```python
from build123d import *

# Parameters (mm, degrees)
BOSS_EXTRUDE1_DEPTH = 2
BOSS_EXTRUDE2_DEPTH = 38
MANUAL_FILLET_DEPTH = 38
SKETCH7_R           = 1.399999999999996
SKETCH7_R_2         = 1.4
SKETCH7_R_3         = 1.3999999999999992
SKETCH7_R_4         = 1.4000000000000026
BOTTOM_SCREWS_DEPTH = 9
LEFT_SCREWS_REACH   = 212.024
SKETCH8_R           = 1.6000000000000127
SKETCH8_R_2         = 1.600000000000008
RIGHT_SCREWS_REACH  = 212.024
SKETCH9_R           = 1.6000000000000127
SKETCH9_R_2         = 1.600000000000007
BOSS_EXTRUDE3_DEPTH = 15
CUT_EXTRUDE1_REACH  = 220.907
SKETCH10_R          = 17.50000000000029
SKETCH10_R_2        = 1.6000000000000194
SKETCH10_R_3        = 1.5999999999999908
CUT_EXTRUDE2_REACH  = 220.907
SKETCH11_R          = 17.500000000000004
SKETCH11_R_2        = 1.600000000000006
SKETCH11_R_3        = 1.5999999999999974
FILLET1_R           = 2


with BuildPart() as part:
    # Sketch2 → Boss-Extrude1 (new body)
    with BuildSketch(Plane.XY):
        Polygon((-113.14018169510446, 0), (113.14018169510446, 2.771e-14), (118.50513169510454, -9.292365980066561), (113.30897927239795, -12.292365980066618), (109.67608007996674, -5.999999999999973), (-109.67608007996674, -6), (-113.30897927239795, -12.292365980066647), (-118.50513169510454, -9.292365980066593), align=None)
    extrude(amount=BOSS_EXTRUDE1_DEPTH)

    # Sketch2<3> → Boss-Extrude2 (add)
    with BuildSketch(Plane.XY):
        Polygon((-113.14018169510446, 0), (113.14018169510446, 2.771e-14), (118.50513169510454, -9.292365980066561), (113.30897927239795, -12.292365980066618), (109.67608007996674, -5.999999999999973), (-109.67608007996674, -6), (-113.30897927239795, -12.292365980066647), (-118.50513169510454, -9.292365980066593), align=None)
    extrude(amount=BOSS_EXTRUDE2_DEPTH)

    # Sketch6 → Manual fillet (add)
    with BuildSketch(Plane(origin=(0, 0, 0), x_dir=(-1, 0, 0), z_dir=(0, 0, -1))):
        with BuildLine():
            Line((-114.87223250267334, -2.99999999999992), (-104.47992765725986, 15.00000000000004))
            ThreePointArc((-104.47992765725986, 15.00000000000004), (-104.47992765725994, 5.00000000000003), (-95.81967361941555, -2.602e-14))
            Line((-95.81967361941555, -2.602e-14), (95.81967361941547, -1.73e-15))
            ThreePointArc((95.81967361941547, -1.73e-15), (104.47992765725988, 5.00000000000004), (104.47992765725981, 15.000000000000083))
            Line((104.47992765725981, 15.000000000000083), (114.87223250267334, -2.999999999999949))
            Line((114.87223250267334, -2.999999999999949), (109.67608007996674, -6))
            Line((109.67608007996674, -6), (-109.67608007996674, -5.999999999999973))
            Line((-109.67608007996674, -5.999999999999973), (-114.87223250267334, -2.99999999999992))
        make_face()
    extrude(amount=-MANUAL_FILLET_DEPTH)

    # Sketch7 → Bottom screws (cut)
    with BuildSketch(Plane.XY):
        with Locations((57.436116251336735, -3.0000000000000004)):
            Circle(SKETCH7_R)
        with Locations((-1.25e-15, -3.0000000000000004)):
            Circle(SKETCH7_R_2)
        with Locations((-57.436116251336564, -3.0000000000000004)):
            Circle(SKETCH7_R)
        with Locations((-28.718058125668286, -3.000000000000001)):
            Circle(SKETCH7_R_3)
        with Locations((28.718058125668367, -3.000000000000001)):
            Circle(SKETCH7_R_3)
        with Locations((-86.15417437700485, -3.000000000000001)):
            Circle(SKETCH7_R_4)
        with Locations((86.15417437700509, -3.000000000000001)):
            Circle(SKETCH7_R_4)
    extrude(amount=BOTTOM_SCREWS_DEPTH, mode=Mode.SUBTRACT)

    # Sketch8 → Left screws (cut, up to next)
    with BuildSketch(Plane(origin=(-79.65898384862079, 45.991135768374306, 0), x_dir=(0, 0, -1), z_dir=(0.8660254037844329, -0.5000000000000101, 0)), mode=Mode.PRIVATE) as left_screws_sk1:
        with Locations(Location((-20, -63.66709165512205, 0), (0, 0, 90))):
            Circle(SKETCH8_R)
    left_screws_tool1 = extrude(left_screws_sk1.sketch, amount=-LEFT_SCREWS_REACH, mode=Mode.PRIVATE) & part.part
    # Sketch8 → Left screws (cut, up to next)
    with BuildSketch(Plane(origin=(-79.65898384862079, 45.991135768374306, 0), x_dir=(0, 0, -1), z_dir=(0.8660254037844329, -0.5000000000000101, 0)), mode=Mode.PRIVATE) as left_screws_sk2:
        with Locations(Location((-4, -63.66709165512205, 0), (0, 0, 90))):
            Circle(SKETCH8_R_2)
    left_screws_tool2 = extrude(left_screws_sk2.sketch, amount=-LEFT_SCREWS_REACH, mode=Mode.PRIVATE) & part.part
    add(left_screws_tool1.solids().sort_by_distance((-111.49253, -9.146183, 20))[0], mode=Mode.SUBTRACT)
    add(left_screws_tool2.solids().sort_by_distance((-111.49253, -9.146183, 4))[0], mode=Mode.SUBTRACT)

    # Sketch9 → Right screws (cut, up to next)
    with BuildSketch(Plane(origin=(79.6589838486208, 45.99113576837435, 0), x_dir=(0, 0, 1), z_dir=(-0.8660254037844329, -0.5000000000000101, 0)), mode=Mode.PRIVATE) as right_screws_sk1:
        with Locations(Location((20, -63.66709165512205, 0), (0, 0, 270))):
            Circle(SKETCH9_R)
    right_screws_tool1 = extrude(right_screws_sk1.sketch, amount=-RIGHT_SCREWS_REACH, mode=Mode.PRIVATE) & part.part
    # Sketch9 → Right screws (cut, up to next)
    with BuildSketch(Plane(origin=(79.6589838486208, 45.99113576837435, 0), x_dir=(0, 0, 1), z_dir=(-0.8660254037844329, -0.5000000000000101, 0)), mode=Mode.PRIVATE) as right_screws_sk2:
        with Locations(Location((4, -63.66709165512205, 0), (0, 0, 270))):
            Circle(SKETCH9_R_2)
    right_screws_tool2 = extrude(right_screws_sk2.sketch, amount=-RIGHT_SCREWS_REACH, mode=Mode.PRIVATE) & part.part
    add(right_screws_tool1.solids().sort_by_distance((111.49253, -9.146183, 20))[0], mode=Mode.SUBTRACT)
    add(right_screws_tool2.solids().sort_by_distance((111.49253, -9.146183, 4))[0], mode=Mode.SUBTRACT)

    # Sketch12 → Boss-Extrude3 (add)
    with BuildSketch(Plane.XY.offset(38.000000000000064)):
        with BuildLine():
            Line((103.86635092950917, 4.062746066806283), (113.30897927239795, -12.292365980066622))
            Line((113.30897927239795, -12.292365980066622), (118.50513169510454, -9.292365980066565))
            Line((118.50513169510454, -9.292365980066565), (104.47992765725988, 15.00000000000004))
            ThreePointArc((104.47992765725988, 15.00000000000004), (105.80397478003607, 9.439883642417866), (103.86635092950917, 4.062746066806283))
        make_face()
        with BuildLine():
            Line((-104.47992765725981, 15.000000000000082), (-118.50513169510454, -9.292365980066597))
            Line((-118.50513169510454, -9.292365980066597), (-113.30897927239795, -12.29236598006665))
            Line((-113.30897927239795, -12.29236598006665), (-103.86635092950914, 4.062746066806313))
            ThreePointArc((-103.86635092950914, 4.062746066806313), (-105.80397478003603, 9.439883642417914), (-104.47992765725981, 15.000000000000082))
        make_face()
    extrude(amount=BOSS_EXTRUDE3_DEPTH)

    # Sketch10 → Cut-Extrude1 (cut, up to next)
    with BuildSketch(Plane(origin=(84.85513627132735, 48.991135768374356, 0), x_dir=(0, 0, -1), z_dir=(0.8660254037844342, 0.500000000000008, 0)), mode=Mode.PRIVATE) as cut_extrude1_sk1:
        with Locations((-38.000000000000085, -76.19999084755334)):
            Circle(SKETCH10_R)
    cut_extrude1_tool1 = extrude(cut_extrude1_sk1.sketch, amount=-CUT_EXTRUDE1_REACH, mode=Mode.PRIVATE) & part.part
    # Sketch10 → Cut-Extrude1 (cut, up to next)
    with BuildSketch(Plane(origin=(84.85513627132735, 48.991135768374356, 0), x_dir=(0, 0, -1), z_dir=(0.8660254037844342, 0.500000000000008, 0)), mode=Mode.PRIVATE) as cut_extrude1_sk2:
        with Locations(Location((-43.99999999999998, -53.69999084755312, 0), (0, 0, 90))):
            Circle(SKETCH10_R_2)
    cut_extrude1_tool2 = extrude(cut_extrude1_sk2.sketch, amount=-CUT_EXTRUDE1_REACH, mode=Mode.PRIVATE) & part.part
    # Sketch10 → Cut-Extrude1 (cut, up to next)
    with BuildSketch(Plane(origin=(84.85513627132735, 48.991135768374356, 0), x_dir=(0, 0, -1), z_dir=(0.8660254037844342, 0.500000000000008, 0)), mode=Mode.PRIVATE) as cut_extrude1_sk3:
        with Locations(Location((-49.99999999999997, -53.69999084755311, 0), (0, 0, 90))):
            Circle(SKETCH10_R_3)
    cut_extrude1_tool3 = extrude(cut_extrude1_sk3.sketch, amount=-CUT_EXTRUDE1_REACH, mode=Mode.PRIVATE) & part.part
    add(cut_extrude1_tool1.solids().sort_by_distance((122.955132, -16.999992, 38))[0], mode=Mode.SUBTRACT)
    add(cut_extrude1_tool2.solids().sort_by_distance((111.705132, 2.48558, 44))[0], mode=Mode.SUBTRACT)
    add(cut_extrude1_tool3.solids().sort_by_distance((111.705132, 2.48558, 50))[0], mode=Mode.SUBTRACT)

    # Sketch11 → Cut-Extrude2 (cut, up to next)
    with BuildSketch(Plane(origin=(-84.85513627132738, 48.99113576837434, 0), x_dir=(0, 0, 1), z_dir=(-0.8660254037844335, 0.500000000000009, 0)), mode=Mode.PRIVATE) as cut_extrude2_sk1:
        with Locations((38.000000000000085, -76.19999084755318)):
            Circle(SKETCH11_R)
    cut_extrude2_tool1 = extrude(cut_extrude2_sk1.sketch, amount=-CUT_EXTRUDE2_REACH, mode=Mode.PRIVATE) & part.part
    # Sketch11 → Cut-Extrude2 (cut, up to next)
    with BuildSketch(Plane(origin=(-84.85513627132738, 48.99113576837434, 0), x_dir=(0, 0, 1), z_dir=(-0.8660254037844335, 0.500000000000009, 0)), mode=Mode.PRIVATE) as cut_extrude2_sk2:
        with Locations(Location((50.00000000000008, -53.699990847553025, 0), (0, 0, 270))):
            Circle(SKETCH11_R_2)
    cut_extrude2_tool2 = extrude(cut_extrude2_sk2.sketch, amount=-CUT_EXTRUDE2_REACH, mode=Mode.PRIVATE) & part.part
    # Sketch11 → Cut-Extrude2 (cut, up to next)
    with BuildSketch(Plane(origin=(-84.85513627132738, 48.99113576837434, 0), x_dir=(0, 0, 1), z_dir=(-0.8660254037844335, 0.500000000000009, 0)), mode=Mode.PRIVATE) as cut_extrude2_sk3:
        with Locations(Location((44.00000000000008, -53.699990847553025, 0), (0, 0, 270))):
            Circle(SKETCH11_R_3)
    cut_extrude2_tool3 = extrude(cut_extrude2_sk3.sketch, amount=-CUT_EXTRUDE2_REACH, mode=Mode.PRIVATE) & part.part
    add(cut_extrude2_tool1.solids().sort_by_distance((-122.955132, -16.999992, 38))[0], mode=Mode.SUBTRACT)
    add(cut_extrude2_tool2.solids().sort_by_distance((-111.705132, 2.48558, 50))[0], mode=Mode.SUBTRACT)
    add(cut_extrude2_tool3.solids().sort_by_distance((-111.705132, 2.48558, 44))[0], mode=Mode.SUBTRACT)

    # Fillet1
    fillet1_edges = [part.edges().sort_by_distance(p)[0] for p in [
        (106.4376651009535, -0.3909007203570517, 38.000000000000064),
        (-106.43766510095352, -0.3909007203571352, 38.000000000000064),
    ]]
    fillet(fillet1_edges, radius=FILLET1_R)


solid = part.part
```
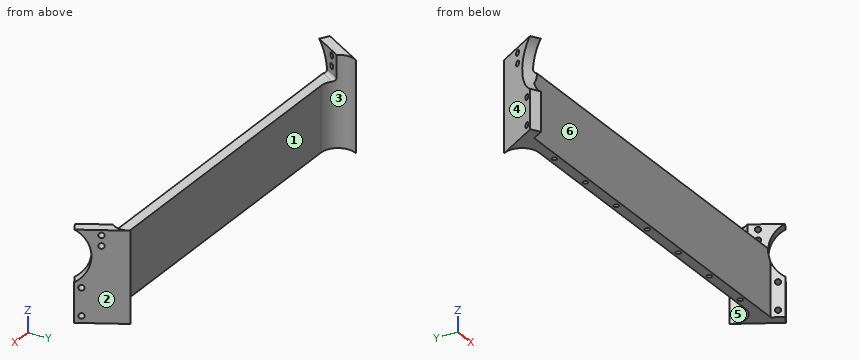
Work out the finished part from the listing and answer in its coordinate system (mm). Face numbers are marked on the shaded views. A direction names the side the tool comes from. Round coordinates to 2 decimals unless told otherwise and drop trailing zeros. Write each loop counter-clockwise with the first axis right and the second up, starting at its lowest first coordinate (ties: lowest second). Pieces come first, ordered by that corner, then holes.
1) A cutting plane is placed at C-C on z = 35. Determine the outline of the cut face in (x, y).
2) Consider probe 1 along Y at (x, z) = (0, 5); probe 2 along Y at (x, z) = (86.5, 26); probe 3 along X at (y, z) = (10.25, 27). Determine where each line is inside the solid, lowest interval first.
3) A cutting plane is placed at B-B on x = -9. Determine the outline of the cut face in (y, z), and give its area (3 significant figures).
4) Which of the six approach directions +Z, -Z, +X, -X, +Y, -Y give full straight-line access (tool end or side, diameter ignored) to the marked faces 1 and 2?
5) A cutting plane is placed at A-A on z = 15.5. Determine the outline of the cut face in (x, y), and give its area (3 significant figures).
6) Determine the mould class of the marked faces 3, 4, 5 and 6 for opening direction Y: pulls with the +Y half, pulls with the -Y half, needs draft (parallel to the pull), parting line crosses it, or undercut.
7) Flat-ended cylindrical pins translate along their axes: P1, Ø12, axis at y = 9, z = 27.5, coming from the +X side; P2, Ø1.5, axis at x = -39, z = 21.5, coming from the -Y side; P3, Ø1.7, axis at x = 57.44, y = -3, coming from the -Z side; P4, Ø3, axis at x = -57.5, y = -8, coming from the -Z side. Find the tip coordinate at first contact, or state that the pin passes through.
Entries:
1. outline: (-114.33, -2.07) - (-107.53, -6) - (107.53, -6) - (114.33, -2.07) - (104.48, 15) arc R10 cw to (95.82, 0) - (-95.82, 0) arc R10 cw to (-104.48, 15) - close
2. probe 1: y = -6 to -4.4, -1.6 to 0
2. probe 2: y = -6 to 0
2. probe 3: x = -107.22 to -105.82, 105.82 to 107.22
3. outline: (-6, 0) - (0, 0) - (0, 38) - (-6, 38) - close
3. area: 228 mm2
4. face 1: +Z, -Z, +Y
4. face 2: +Z, -Z, +X, +Y
5. outline: (-118.51, -9.29) - (-113.31, -12.29) - (-109.68, -6) - (109.68, -6) - (113.31, -12.29) - (118.51, -9.29) - (104.48, 15) arc R10 cw to (95.82, 0) - (-95.82, 0) arc R10 cw to (-104.48, 15) - close
5. area: 1,580 mm2
6. face 3: undercut
6. face 4: pulls with the +Y half
6. face 5: undercut
6. face 6: pulls with the -Y half
7. P1: stops at x = 111.41
7. P2: stops at y = -6
7. P3: stops at z = 9
7. P4: passes through
